Source: CAD feature listing. Evaluate the final solid. Frame: model axes, mm. A direction names the side the tool comes from. Give positions to 0.01 mm unless a question says otherwise; leave off trailing zeros. Order: outer loops, then holes, each group sorted by start corner. A loop starts at its lowest first (then second) coordinate and runs counter-clockwise, first axis right, second up. Notation, with made-up numbers: M 19,30 L 26,30 A27 cw 26,54 Z; hole C 27.5,-3 d10. An arc over 180 degrees is marked long. Answer in a Markdown table with one row per item. Add a question column.
(1) Section query D-D, the plane y = -5.25. Return loops of the section in (x, z), plus the area to 3 significant figures.
(2) Material intervals for line 1 along X through (y, z) = (1.5, 13.25); line 2 along Z through (x, y) = (-4.5, 3), sorted ascending.
(3) Section query C-C, the plane x = 0. Return loops of the section in (y, z), plus the area to 3 significant figures.
(4) Section query B-B, the plane z = 3. Return loops of the section in (x, y), plus the area to 3 significant figures.
(5) Pin query (flat end, axial travel): P1, Ø1.5, axis at y = 4.5, z = 8.5, coming from the -X side; P2, Ø8, axis at x = -5, z = 12, coming from the -Y side; P3, Ø5, axis at y = -4, z = 7, coming from the +X side; P4, Ø5, axis at x = -0.5, z = 6.5, coming from the +Y side. Return the tip coordinate at first contact, or that it passes through.
(6) Set-up query: faces 1 (the face through (-0.325, 6.268, 13.464)), 2 (the face through (-0.325, -6.232, 13.464)), 3 (the face through (-6.232, 0.195, 1.513)), 4 (the face through (6.268, 0.195, 1.513)). Return all of +Z, -Z, +X, -X, +Y, -Y with unobstructed straight access to the full face (end or side cutting, diameter ignored); none if empty.
(7) Section query A-A, the plane y = 0. Return loops of the section in (x, z).
from build123d import *

# Parameters (mm, degrees)
SKETCH1_W           = 10
SKETCH1_H           = 10
BOSS_EXTRUDE1_DEPTH = 15
SKETCH3_R           = 1.5
BOSS_EXTRUDE2_DEPTH = 7.5
SKETCH4_R           = 1.5
BOSS_EXTRUDE3_DEPTH = 7.5


with BuildPart() as part:
    # Sketch1 → Boss-Extrude1 (new body)
    with BuildSketch(Plane.XY):
        Rectangle(SKETCH1_W, SKETCH1_H)
    extrude(amount=BOSS_EXTRUDE1_DEPTH)

    # Sketch2 → Cut-Revolve1 (revolve, cut)
    with BuildSketch(Plane(origin=(0, 0, 0), x_dir=(1, 0, 0), z_dir=(0, 1, 0)), mode=Mode.PRIVATE) as cut_revolve1_sk:
        Polygon((-4.75, 0), (-15.04, 0), (-15.04, -15), (-4.75, -15), (-12.5, -10.525535414), (-12.5, -4.474464586), align=None)
    revolve(cut_revolve1_sk.sketch.rotate(Axis((0, 0, 15.75), (0, 0, -1)), 44.999991596), axis=Axis((0, 0, 15.75), (0, 0, -1)), mode=Mode.SUBTRACT)

    # Sketch3 → Boss-Extrude2 (add, symmetric)
    with BuildSketch(Plane(origin=(0, 0, 0), x_dir=(1, 0, 0), z_dir=(0, 1, 0))):
        with Locations((0, -12)):
            Circle(SKETCH3_R)
    extrude(amount=BOSS_EXTRUDE2_DEPTH, both=True)

    # Sketch4 → Boss-Extrude3 (add, symmetric)
    with BuildSketch(Plane(origin=(0, 0, 0), x_dir=(0, 0, -1), z_dir=(1, 0, 0))):
        with Locations(Location((-3, 0, 0), (0, 0, 270))):
            Circle(SKETCH4_R)
    extrude(amount=BOSS_EXTRUDE3_DEPTH, both=True)


solid = part.part
Values follow:
| question | item | result |
|---|---|---|
| 1 | outline | C 0,12 d3 |
| 1 | area | 7.07 mm² |
| 2 | line 1 | x = -5 to 5 |
| 2 | line 2 | z = 0.38 to 14.62 |
| 3 | outline | M -7.5,10.5 L -5,10.5 L -5,0.14 L -4.75,0 L 4.75,0 L 5,0.14 L 5,10.5 L 7.5,10.5 L 7.5,13.5 L 5,13.5 L 5,14.86 L 4.75,15 L -4.75,15 L -5,14.86 L -5,13.5 L -7.5,13.5 Z |
| 3 | area | 165 mm² |
| 4 | outline | M -7.5,-1.5 L -5,-1.5 L -5,-5 L 5,-5 L 5,-1.5 L 7.5,-1.5 L 7.5,1.5 L 5,1.5 L 5,5 L -5,5 L -5,1.5 L -7.5,1.5 Z |
| 4 | area | 115 mm² |
| 5 | P1 | stops at x = -5 |
| 5 | P2 | stops at y = -7.5 |
| 5 | P3 | stops at x = 5 |
| 5 | P4 | stops at y = 5 |
| 6 | face 1 | +Y |
| 6 | face 2 | -Y |
| 6 | face 3 | -X |
| 6 | face 4 | +X |
| 7 | outline | M -7.5,1.5 L -5,1.5 L -5,0.14 L -4.75,0 L 4.75,0 L 5,0.14 L 5,1.5 L 7.5,1.5 L 7.5,4.5 L 5,4.5 L 5,14.86 L 4.75,15 L -4.75,15 L -5,14.86 L -5,4.5 L -7.5,4.5 Z |
